Build history of the part. All positions in model axes, mm. A direction names the side the tool comes from. Round coordinates to 2 decimals unless told otherwise and drop trailing zeros. Write each loop counter-clockwise with the first axis right and the second up, starting at its lowest first coordinate (ties: lowest second). Pieces come first, ordered by that corner, then holes. Notation, with made-up numbers: M -17,28 L 9,28 A6 ccw 9,37 Z; hole C 39.5,77.25 d8. An arc over 180 degrees is marked long. Write item = value, one per line. Start each with the question number.
Q1. Band-saw the part on C-C on x = 69.5. Write the cut outline in (y, z), plus the area to 3 significant figures.
Q2. Probe L1, parallel to X at y = -8.25, z = 5.5; L2, parallel to Y at x = 67.5, z = 0.5; L3, parallel to Y at x = 42, z = 0. List the from-to ranges inside material, lowest first.
Q3. Band-saw the part on D-D on x = 54. Write the cut outline in (y, z), plus the area to 3 significant figures.
Q4. Tool access for faces 4 (the flat face through (85, 4, 0)), 5 (the cylindrical face through (7.605, -7.493, -0.33)), 6 (the flat face through (40, 6, 0)), 7 (the cylindrical face through (72.605, -7.493, -0.33)): list every direction of +Z, -Z, +X, -X, +Y, -Y with a clear straight run to the whole face (end or side of a thin tool).
Q5. Drop flat-ended pins along their axis: P1, Ø8, axis at x = 63, z = 7, coming from the +Y side; P2, Ø10, axis at x = 69, y = 7, coming from the +Z side; P3, Ø2, axis at y = 9, z = 4, coming from the +X side; P4, Ø10, axis at x = 23.5, z = 5, coming from the +Y side. Give the stop position or say it passes through.
Q6. Pull direction X, two halves, no side cores. Call faces 1 (the flat face through (30, 8, 0)), 2 (the cylindrical face through (85, -5, 0)), 3 (the flat face through (80, 5, 0)): released by +X, released by -X, zero draft, split by the parting line, or undercut.
Q7. Band-saw the part on B-B on z = 0. Write the cut outline in (x, y).
Q8. Band-saw the part on A-A on y = 0. Write the cut outline in (x, z), plus the area to 3 significant figures.
```python
from build123d import *

# Parameters (mm, degrees)
IZIM3_W               = 20
IZIM3_H               = 8.956518763
IZIM3_W_2             = 16.233107577
IZIM3_H_2             = 7.025571552
KES_EKSTR_ZYON1_DEPTH = 30


with BuildPart() as part:
    # Çizim1 → Döndür2 (revolve)
    with BuildSketch(Plane.XY):
        Polygon((0, 0), (0, 7.5), (15, 7.5), (15, 10), (65, 10), (65, 7.5), (80, 7.5), (80, 5), (90, 5), (90, 0), align=None)
    revolve(axis=Axis((90, 0, 0), (-1, 0, 0)))

    # Çizim3 → Kes-Ekstrüzyon1 (cut, symmetric)
    with BuildSketch(Plane.XY):
        with Locations((40, 10.478259381)):
            Rectangle(IZIM3_W, IZIM3_H)
        with Locations((88.116553788, 7.512785776)):
            Rectangle(IZIM3_W_2, IZIM3_H_2)
    extrude(amount=KES_EKSTR_ZYON1_DEPTH, both=True, mode=Mode.SUBTRACT)


solid = part.part
```
Conclusion:
q1.outline = C 0,0 d15
q1.area = 177 mm^2
q2.L1 = 15 to 65
q2.L2 = -7.48 to 7.48
q2.L3 = -10 to 6
q3.outline = C 0,0 d20
q3.area = 314 mm^2
q4.face_4 = +Z, -Z, +X, +Y
q4.face_5 = -X
q4.face_6 = +Z, -Z, +Y
q4.face_7 = +X
q5.P1 = 9.54
q5.P2 = 9.17
q5.P3 = 65
q5.P4 = 10
q6.face_1 = undercut
q6.face_2 = zero draft
q6.face_3 = released by +X
q7.outline = M 0,-7.5 L 15,-7.5 L 15,-10 L 65,-10 L 65,-7.5 L 80,-7.5 L 80,-5 L 90,-5 L 90,4 L 80,4 L 80,7.5 L 65,7.5 L 65,10 L 50,10 L 50,6 L 30,6 L 30,10 L 15,10 L 15,7.5 L 0,7.5 Z
q8.outline = M 0,-7.5 L 15,-7.5 L 15,-10 L 65,-10 L 65,-7.5 L 80,-7.5 L 80,-5 L 90,-5 L 90,5 L 80,5 L 80,7.5 L 65,7.5 L 65,10 L 15,10 L 15,7.5 L 0,7.5 Z
q8.area = 1,550 mm^2
